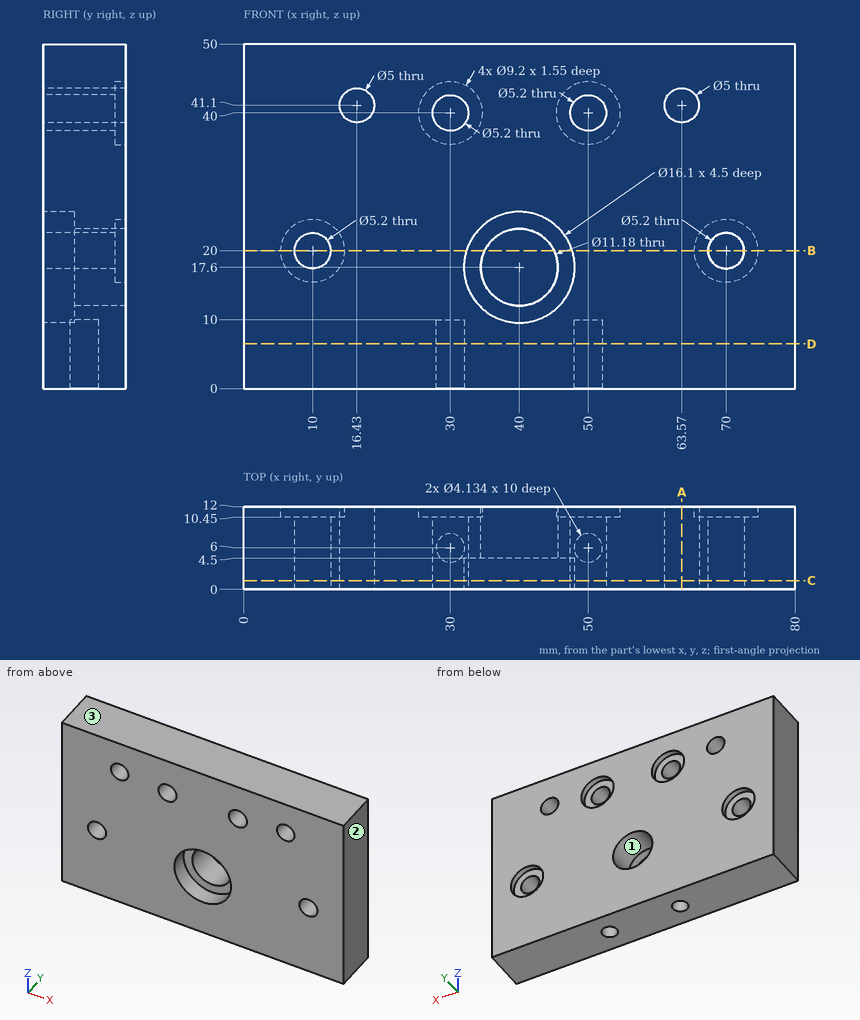
Study the drawing (mm; zero at the part's minimum x, y, z) and answer. Give positions to 0.01 mm unless a question says otherwise; leave off trailing zeros. Loops run counter-clockwise (first coordinate to the right, second up) from the corner with the lowest first, then second, coordinate; pieces in that order, holes last. Notation, with made-up numbers: M 20,5 L 72,5 A10 ccw 72,24 Z; hole C 88.25,39.5 d10. An arc over 180 degrees is marked long. One line per item, written item: value. Start each with the question number.
1. Find section D-D (z = 6.5). Give the vertices of the cut face in (x, y), and give its area (3 significant figures).
2. Find section A-A (x = 63.57). Give the vertices of the cut face in (y, z).
3. Determine the mould class of the marked faces 1, 2 and 3 for opening direction Z: released by +Z, released by -Z, zero draft, split by the parting line, or undercut.
4. Each of these flat-tipped pins is pushed along its axis until it touches: P1, Ø10.5, axis at x = 30, z = 40, coming from the -Y side; P2, Ø13, axis at x = 40, z = 17.6, coming from the -Y side; P3, Ø1.2, axis at x = 50.5, y = 6.5, coming from the -Z side. Where does it stop, or does it pass through?
5. Find section B-B (z = 20). Give the vertices of the cut face in (x, y), and give its area (3 significant figures).
6. Find the intervals of material crossed by probe 1 along Z at (x, y) = (30, 11.25); probe 2 along Z at (x, y) = (10, 11.6); probe 3 along Y at (x, z) = (50, 5), in increasing order.
7. Find section C-C (y = 1.25). Give the vertices of the cut face in (x, z).
Reported:
1. outline: M 0,0 L 80,0 L 80,12 L 0,12 Z; hole C 30,6 d4.13; hole C 50,6 d4.13
1. area: 933 mm²
2. outline: M 0,0 L 12,0 L 12,38.6 L 0,38.6 Z; M 0,43.6 L 12,43.6 L 12,50 L 0,50 Z
3. face 1: undercut
3. face 2: zero draft
3. face 3: released by +Z
4. P1: stops at y = 0
4. P2: stops at y = 4.5
4. P3: stops at z = 10
5. outline: M 0,0 L 7.4,0 L 7.4,10.45 L 5.4,10.45 L 5.4,12 L 0,12 Z; M 12.6,0 L 32.32,0 L 32.32,4.5 L 34.95,4.5 L 34.95,12 L 14.6,12 L 14.6,10.45 L 12.6,10.45 Z; M 45.05,4.5 L 47.68,4.5 L 47.68,0 L 67.4,0 L 67.4,10.45 L 65.4,10.45 L 65.4,12 L 45.05,12 Z; M 72.6,0 L 80,0 L 80,12 L 74.6,12 L 74.6,10.45 L 72.6,10.45 Z
5. area: 678 mm²
6. probe 1: z = 0 to 35.4, 44.6 to 50
6. probe 2: z = 0 to 15.4, 24.6 to 50
6. probe 3: y = 0 to 3.93, 8.07 to 12
7. outline: M 0,0 L 80,0 L 80,50 L 0,50 Z; hole C 10,20 d5.2; hole C 16.43,41.1 d5; hole C 30,40 d5.2; hole C 40,17.6 d16.1; hole C 50,40 d5.2; hole C 63.57,41.1 d5; hole C 70,20 d5.2
